The listing builds one solid part. Answer for the finished solid, in the listing's coordinates (mm). A direction names the side the tool comes from. Round coordinates to 2 decimals unless told otherwise and drop trailing zeros. Write each loop counter-clockwise with the first axis right and the second up, starting at its lowest first coordinate (ties: lowest second). Pieces come first, ordered by that corner, then holes.
(1) A cutting plane is placed at B-B, the plane x = -131. Give the vertices of the cut face in (y, z), and give its area (3 significant figures).
(2) A cutting plane is placed at A-A, the plane y = 172. Give the vertices of the cut face in (x, z), and give its area (3 significant figures).
(3) For faces 4 (the face through (0, 73, 2)), 5 (the face through (23, 63, 2)), 6 (the face through (-192, 195, 2)), 7 (the face through (-193, 175, 2)), determine the directions among +Z, -Z, +X, -X, +Y, -Y from which every point of the face is accessible in a straight line to the end or side of a thin tool.
(4) Each of these flat-tipped pins is pushed along its axis until it touches: pin 1 Ø0.9 at (y, z) = (21, 3) entering from +X; pin 2 Ø1.4 at (x, z) = (12, 1.5) entering from +Y; pin 3 Ø1.5 at (x, z) = (22, 3.5) entering from -Y. Where does it stop, or does it pass through?
(5) The mould has two halves that part along Y. Classify faces 1 (the face through (-182, 23.5, 2)), 2 (the face through (-190, 10, 2)), 3 (the face through (8, 0, 2)): +Y half, -Y half, draft (parallel to the pull), parting line (faces both ways), or undercut.
(6) Find the intervals of material crossed by probe 1 along Y at (x, z) = (-24, 4.4); probe 2 along X at (y, z) = (17.5, 3); probe 3 along Y at (x, z) = (-126.5, 2.85), in increasing order.
from build123d import *

# Parameters (mm, degrees)
BOSS_EXTRU_1_DEPTH = 5
CONG_1_R           = 5


with BuildPart() as part:
    # Esquisse1 → Boss.-Extru.1 (new body)
    with BuildSketch(Plane.XY):
        Polygon((0, 0), (20, 0), (20, 13), (25, 13), (25, 18), (20, 18), (20, 21.5), (17, 21.5), (17, 20.4), (14.7, 20.4), (14.7, 21.5), (10, 21.5), (10, 24.5), (14.7, 24.5), (14.7, 25.6), (17, 25.6), (17, 24.5), (20, 24.5), (20, 28), (25, 28), (25, 33), (20, 33), (20, 43), (25, 43), (25, 48), (20, 48), (20, 51.5), (17, 51.5), (17, 50.4), (14.7, 50.4), (14.7, 51.5), (10, 51.5), (10, 54.5), (14.7, 54.5), (14.7, 55.6), (17, 55.6), (17, 54.5), (20, 54.5), (20, 58), (25, 58), (25, 63), (20, 63), (20, 71), (15, 71), (15, 76), (10, 76), (10, 71), (6.5, 71), (6.5, 68), (7.6, 68), (7.6, 65.7), (6.5, 65.7), (6.5, 61), (3.5, 61), (3.5, 65.7), (2.4, 65.7), (2.4, 68), (3.5, 68), (3.5, 71), (0, 71), (0, 76), (-5, 76), (-5, 71), (-40, 71), (-150, 210), (-190, 210), (-190, 195), (-195, 195), (-195, 190), (-190, 190), (-190, 186.5), (-187, 186.5), (-187, 187.6), (-184.7, 187.6), (-184.7, 186.5), (-180, 186.5), (-180, 183.5), (-184.7, 183.5), (-184.7, 182.4), (-187, 182.4), (-187, 183.5), (-190, 183.5), (-190, 180), (-195, 180), (-195, 175), (-190, 175), (-190, 35), (-195, 35), (-195, 30), (-190, 30), (-190, 26.5), (-187, 26.5), (-187, 27.6), (-184.7, 27.6), (-184.7, 26.5), (-180, 26.5), (-180, 23.5), (-184.7, 23.5), (-184.7, 22.4), (-187, 22.4), (-187, 23.5), (-190, 23.5), (-190, 20), (-195, 20), (-195, 15), (-190, 15), (-190, 0), (-170, 0), (-150, 20), (-20, 20), align=None)
    extrude(amount=BOSS_EXTRU_1_DEPTH)

    # Congé1
    cong_1_edges = [part.edges().sort_by_distance(p)[0] for p in [
        (20, 0, 2.5),
        (0, 0, 2.5),
        (-20, 20, 2.5),
        (-150, 20, 2.5),
        (-170, 0, 2.5),
        (-190, 0, 2.5),
        (-190, 210, 2.5),
        (-150, 210, 2.5),
        (-40, 71, 2.5),
    ]]
    fillet(cong_1_edges, radius=CONG_1_R)


solid = part.part
Solutions:
1. outline: (20, 0) - (185.99, 0) - (185.99, 5) - (20, 5) - close
1. area: 830 mm2
2. outline: (-190, 0) - (-119.93, 0) - (-119.93, 5) - (-190, 5) - close
2. area: 350 mm2
3. face 4: +Z, -Z, +Y
3. face 5: +Z, -Z, +X, +Y
3. face 6: +Z, -Z, -X, +Y
3. face 7: +Z, -Z, -X
4. pin 1: stops at x = 20
4. pin 2: stops at y = 76
4. pin 3: stops at y = 13
5. face 1: undercut
5. face 2: draft
5. face 3: -Y half
6. probe 1: y = 20 to 71
6. probe 2: x = -195 to -152.5, -17.5 to 25
6. probe 3: y = 20 to 180.3
